Check sheet for the modelled part. Datum: model origin and axes. Units: mm. A direction names the side the tool comes from. Coordinates: 2 decimals unless noted, no trailing zeros. Write each loop counter-clockwise with the first axis right and the second up, starting at its lowest first coordinate (ties: lowest second). Pieces come first, ordered by that corner, then holes. Notation, with made-up numbers: (17.25, -29.5) -> (75.25, -29.5) arc R18 ccw to (75.25, -21.5) -> close; hole circle Ø11 at (34.25, 53.25). An arc over 180 degrees is marked (long way). Put each result on its own line as item: value.
```python
from build123d import *

# Parameters (mm, degrees)
SKETCH1_R           = 19.05
BOSS_EXTRUDE1_DEPTH = 3.81


with BuildPart() as part:
    # Sketch1 → Boss-Extrude1 (new body)
    with BuildSketch(Plane.XY):
        with Locations(Location((0, 0, 0), (0, 0, 180))):
            Circle(SKETCH1_R)
        with BuildLine():
            Line((1.118033989, 1), (-1.118033989, 1))
            ThreePointArc((-1.118033989, 1), (0, -1.5), (1.118033989, 1))
        make_face(mode=Mode.SUBTRACT)
        with BuildLine():
            Line((13.829158979, 1.016666667), (11.570841021, 1.016666667))
            ThreePointArc((11.570841021, 1.016666667), (12.7, -1.533333333), (13.829158979, 1.016666667))
        make_face(mode=Mode.SUBTRACT)
        with BuildLine():
            Line((5.942864327, 12.455213271), (4.802688902, 10.480371506))
            ThreePointArc((4.802688902, 10.480371506), (7.624442664, 10.167792388), (5.942864327, 12.455213271))
        make_face(mode=Mode.SUBTRACT)
        with BuildLine():
            Line((-7.917318674, 11.327860481), (-6.76623223, 9.334120277))
            ThreePointArc((-6.76623223, 9.334120277), (-5.046808132, 11.655990379), (-7.917318674, 11.327860481))
        make_face(mode=Mode.SUBTRACT)
        with BuildLine():
            Line((-13.861895004, -1.256937352), (-11.538104996, -1.256937352))
            ThreePointArc((-11.538104996, -1.256937352), (-12.7, 1.443062648), (-13.861895004, -1.256937352))
        make_face(mode=Mode.SUBTRACT)
        with BuildLine():
            Line((-5.915422385, -12.698362956), (-4.742818445, -10.667353355))
            ThreePointArc((-4.742818445, -10.667353355), (-7.710690276, -10.307858156), (-5.915422385, -12.698362956))
        make_face(mode=Mode.SUBTRACT)
        with BuildLine():
            Line((7.977039629, -11.520341387), (6.793823672, -9.470951234))
            ThreePointArc((6.793823672, -9.470951234), (4.96056052, -11.89564631), (7.977039629, -11.520341387))
        make_face(mode=Mode.SUBTRACT)
    extrude(amount=BOSS_EXTRUDE1_DEPTH)


solid = part.part
```
Q1. Cross-section at C-C (y = 10). Record the cut outline in (x, z).
Recorded:
outline: (-16.21, 0) -> (-7.15, 0) -> (-7.15, 3.81) -> (-16.21, 3.81) -> close; (-5.1, 0) -> (5.05, 0) -> (5.05, 3.81) -> (-5.1, 3.81) -> close; (7.51, 0) -> (16.21, 0) -> (16.21, 3.81) -> (7.51, 3.81) -> close
Q2. Tool access check on faces 1 (the flat face through (-7.35, 10.345, 1.878)), 2 (the flat face through (-4, 0, 3.81)). Record the directions out of +Z, -Z, +X, -X, +Y, -Y that give a thin tool (end or side, any length) a straight path to the whole face; none if there is none.
Recorded:
face 1: +Z, -Z
face 2: +Z, +X, -X, +Y, -Y
Q3. Cross-section at B-B (z = 1.5). State how many separate pieces and enclosed holes the cut face has, plus the area to 3 significant figures.
Recorded:
separate pieces: 1
enclosed holes: 7
area: 1,090 mm2
Q4. Depth check by flat-ended pin: P1, Ø1.5, axis at x = -14.5, z = 2, coming from the -Y side; P2, Ø4.5, axis at x = 6.39, y = -11.07, coming from the -Z side; P3, Ø0.7, axis at x = 0, z = 2.5, coming from the -Y side; P4, Ø1.2, axis at x = -12, z = 1.5, coming from the +Y side. Enter the tip coordinate at first touch or a pass-through.
Recorded:
P1: stops at y = -13.18
P2: stops at z = 0
P3: stops at y = -19.05
P4: stops at y = 15.26
Q5. Mould release check, pull along Y, two halves, no side actions. Record for faces 3 (the cylindrical face through (12.651, -1.533, 1.878)), 4 (the flat face through (-4, 0, 0)), 5 (the cylindrical face through (4.13, 18.597, 1.878)): released by +Y, released by -Y, zero draft, split by the parting line, or undercut.
Recorded:
face 3: undercut
face 4: zero draft
face 5: split by the parting line
Q6. Cross-section at A-A (x = 0). Record the cut outline in (y, z), plus the area to 3 significant figures.
Recorded:
outline: (-19.05, 0) -> (-1.5, 0) -> (-1.5, 3.81) -> (-19.05, 3.81) -> close; (1, 0) -> (19.05, 0) -> (19.05, 3.81) -> (1, 3.81) -> close
area: 136 mm2
Q7. Cross-section at D-D (x = 12.7). Record the cut outline in (y, z), plus the area to 3 significant figures.
Recorded:
outline: (-14.2, 0) -> (-1.53, 0) -> (-1.53, 3.81) -> (-14.2, 3.81) -> close; (1.02, 0) -> (14.2, 0) -> (14.2, 3.81) -> (1.02, 3.81) -> close
area: 98.5 mm2
Q8. Material ranges on line 1 along X through (y, z) = (-10, 1.15); line 2 along Y through (x, z) = (5, 3.45); line 3 along Y through (x, z) = (-6, 1.4), recorded low to high.
Recorded:
line 1: x = -16.21 to -7.48, -5.13 to 5.13, 7.1 to 16.21
line 2: y = -18.38 to -11.96, -10.18 to 10.07, 10.82 to 18.38
line 3: y = -18.08 to -12.72, -9.52 to 9.35, 12.39 to 18.08
